Here's how the part is built. I have some questions about the finished solid (model axes, mm). A direction names the side the tool comes from. Give positions to 0.01 mm unless a question says otherwise; leave off trailing zeros. Loops run counter-clockwise (first coordinate to the right, second up) from the corner with the lowest first, then second, coordinate; pieces in that order, holes last. Notation, with made-up numbers: M 46,-6 L 102,-6 A14 cw 102,19 Z; hole C -10.5,20.5 d2. An arc over 180 degrees is marked long. Answer as CSV lines item,"result". Start each with the question number.
Item 1: For faces 1 (the cylindrical face through (-7.509, 30.073, -23.846)), 2 (the flat face through (7.5, 56, -23)), 3 (the flat face through (-24, 57, 0)), which set-ups out of +Z, -Z, +X, -X, +Y, -Y let a thin tool reach every point of the face, with its end or its side?
Item 2: I want a section at B-B on z = -12. List the corners of the cut face in (x, y) for me.
Item 3: I want a section at D-D on z = 0. List the corners of the cut face in (x, y) for me, plus the area to 3 significant figures.
Item 4: I want a section at A-A on x = 0. List the corners of the cut face in (y, z) for me, plus the area to 3 significant figures.
Item 5: If we mould it in two halves opening along Y, with no side actions, what happens to faces 4 (the flat face through (22.1, 0, -7.3)), 5 (the flat face through (-23, 56, -7.5)), 6 (the flat face through (0, 55, -24))? For each: released by +Y, released by -Y, zero draft, split by the parting line, or undercut.
Item 6: I want a section at C-C on x = 20.5. List the corners of the cut face in (y, z) for me, plus the area to 3 significant figures.
Item 7: If I drill on line 1 along X through (y, z) = (18, 0); line 2 along X through (y, z) = (45.5, -18); line 3 along Z through (x, y) = (2, 27), over which ranges is the centre line in solid material (lowest first)? Write a range as from..to.
Item 8: Will these pins go through, and if not, where does the flat tip stop? P1, Ø1, axis at x = 24, z = -0.5, coming from the -Y side; P2, Ø6, axis at x = -13.5, z = 12, coming from the +Y side; P3, Ø1, axis at y = 56.5, z = 23, coming from the -X side; P4, Ø2, axis at x = -22.5, y = 55.5, coming from the +Z side.
from build123d import *

# Parameters (mm, degrees)
SKETCH1_R           = 25
SKETCH1_R_2         = 23
BOSS_EXTRUDE1_DEPTH = 61
SKETCH2_W           = 15
SKETCH2_H           = 2
CUT_EXTRUDE2_DEPTH  = 26
CIRPATTERN1_COUNT   = 4


with BuildPart() as part:
    # Sketch1 → Boss-Extrude1 (new body)
    with BuildSketch(Plane(origin=(0, 0, 0), x_dir=(1, 0, 0), z_dir=(0, 1, 0))):
        with Locations(Location((0, 0, 0), (0, 0, 90))):
            Circle(SKETCH1_R)
        with Locations(Location((0, 0, 0), (0, 0, 90))):
            Circle(SKETCH1_R_2, mode=Mode.SUBTRACT)
    extrude(amount=BOSS_EXTRUDE1_DEPTH)

    # Sketch2 → Cut-Extrude2 (cut)
    with BuildSketch(Plane.XY):
        with Locations((0, 56)):
            Rectangle(SKETCH2_W, SKETCH2_H)
    cut_extrude2 = extrude(amount=-CUT_EXTRUDE2_DEPTH, mode=Mode.SUBTRACT)

    # CirPattern1: Cut-Extrude2 ×4 about axis
    cirpattern1_axis = Axis((0, 0, 0), (0, 1, 0))
    for i in range(1, CIRPATTERN1_COUNT):
        add(cut_extrude2.rotate(cirpattern1_axis, i * 360 / CIRPATTERN1_COUNT), mode=Mode.SUBTRACT)


solid = part.part
Result:
1,face 1,"+Y, -Y"
1,face 2,"+Z, -Z"
1,face 3,"+X, -X"
2,outline,"M -21.93,0 L -19.62,0 L -19.62,61 L -21.93,61 Z; M 19.62,0 L 21.93,0 L 21.93,61 L 19.62,61 Z"
3,outline,"M -25,0 L -23,0 L -23,55 L -25,55 Z; M -25,57 L -23,57 L -23,61 L -25,61 Z; M 23,0 L 25,0 L 25,55 L 23,55 Z; M 23,57 L 25,57 L 25,61 L 23,61 Z"
3,area,"236 mm^2"
4,outline,"M 0,-25 L 55,-25 L 55,-23 L 0,-23 Z; M 0,23 L 55,23 L 55,25 L 0,25 Z; M 57,-25 L 61,-25 L 61,-23 L 57,-23 Z; M 57,23 L 61,23 L 61,25 L 57,25 Z"
4,area,"236 mm^2"
5,face 4,"released by -Y"
5,face 5,"undercut"
5,face 6,"undercut"
6,outline,"M 0,-14.31 L 61,-14.31 L 61,-10.43 L 0,-10.43 Z; M 0,10.43 L 61,10.43 L 61,14.31 L 0,14.31 Z"
6,area,"473 mm^2"
7,line 1,"-25..-23, 23..25"
7,line 2,"-17.35..-14.32, 14.32..17.35"
7,line 3,"-24.92..-22.91, 22.91..24.92"
8,P1,"y = 0"
8,P2,"through"
8,P3,"x = -10.9"
8,P4,"z = 12.76"
